Here's how the part is built. I have some questions about the finished solid (model axes, mm). Coordinates: 2 decimals unless noted, no trailing zeros. Order: outer loops, then holes, each group sorted by start corner. A loop starts at its lowest first (then second) coordinate and runs counter-clockwise, first axis right, second up. Notation, with made-up numbers: (58, 49.5) - (109, 49.5) arc R34 ccw to (109, 86.5) - close; hole circle Ø6 at (40.5, 23.5). An arc over 180 degrees is marked (long way). Answer in a Markdown table with one row per item. Add a question column.
Item 1: I want a section at C-C (z = 10.5). Please give me the cut outline in (x, y), plus the area to 3 significant figures.
Item 2: Will these pins go through, and if not, where does the flat tip stop? pin 1 Ø2 at (x, z) = (-15.5, -20) entering from +Y; pin 2 Ø3 at (x, z) = (-27.5, -8) entering from +Y; pin 3 Ø4 at (x, z) = (-24.5, -24.5) entering from +Y.
Item 3: If I drill on line 1 along Y through (x, z) = (42, -13); line 2 along Y through (x, z) = (-41, -8.5), over which ranges is the centre line in solid material (lowest first)? Write a range as from..to.
Item 4: I want a section at B-B (z = 1.5). Please give me the cut outline in (x, y).
```python
from build123d import *

# Parameters (mm, degrees)
SKETCH1_W           = 130
SKETCH1_H           = 80
BOSS_EXTRUDE1_DEPTH = 60
CHAMFER1_SIZE2      = 80
CHAMFER1_SIZE       = 20


with BuildPart() as part:
    # Sketch1 → Boss-Extrude1 (new body)
    with BuildSketch(Plane(origin=(0, 0, 0), x_dir=(1, 0, 0), z_dir=(0, 1, 0))):
        Rectangle(SKETCH1_W, SKETCH1_H)
    extrude(amount=BOSS_EXTRUDE1_DEPTH)

    # Chamfer1
    chamfer1_edges = [part.edges().sort_by_distance(p)[0] for p in [
        (0, 60, 40),
    ]]
    chamfer1_side = [part.faces().sort_by_distance(p)[0] for p in [
        (0, 59.6, 40),
    ]]
    chamfer(chamfer1_edges, length=CHAMFER1_SIZE - 0.0001, length2=CHAMFER1_SIZE2 - 0.0001, reference=chamfer1_side[0])  # a hair under: the kernel refuses the full size


solid = part.part
```
Values follow:
| question | item | result |
|---|---|---|
| 1 | outline | (-65, 0) - (65, 0) - (65, 47.38) - (-65, 47.38) - close |
| 1 | area | 6,160 mm^2 |
| 2 | pin 1 | stops at y = 55.25 |
| 2 | pin 2 | stops at y = 52.38 |
| 2 | pin 3 | stops at y = 56.63 |
| 3 | line 1 | y = 0..53.25 |
| 3 | line 2 | y = 0..52.13 |
| 4 | outline | (-65, 0) - (65, 0) - (65, 49.63) - (-65, 49.63) - close |
